from build123d import *

# Parameters (mm, degrees)
SKETCH_3_W             = 131
SKETCH_3_H             = 80
EXTRUDE_3_DEPTH        = 5
SKETCH_4_W             = 119
SKETCH_4_H             = 80
EXTRUDE_4_DEPTH        = 6
FILLET_2_R             = 5
CHAMFER_1_SIZE         = 1
CUT_EXTRUDE_1_DEPTH    = 6
FILLET_3_R             = 5
CHAMFER_2_SIZE         = 1
SKETCH_6_R             = 2.2
CUT_EXTRUDE_2_DEPTH    = 11
HOLE_WIZARD_M3_1_D     = 2.5
HOLE_WIZARD_M3_1_DEPTH = 7.5
HOLE_WIZARD_M3_1_TIP   = 0.751075774


with BuildPart() as part:
    # 草图3 → 凸台-拉伸3 (new body)
    with BuildSketch(Plane.XY):
        with Locations((0, -51.5)):
            Rectangle(SKETCH_3_W, SKETCH_3_H)
    extrude(amount=EXTRUDE_3_DEPTH)

    # 草图4 → 凸台-拉伸4 (add)
    with BuildSketch(Plane.XY.offset(5)):
        with Locations((0, -51.5)):
            Rectangle(SKETCH_4_W, SKETCH_4_H)
    extrude(amount=-EXTRUDE_4_DEPTH)

    # 圆角2
    fillet_2_edges = [part.edges().sort_by_distance(p)[0] for p in [
        (-65.5, -11.5, 2.5),
        (65.5, -11.5, 2.5),
        (65.5, -91.5, 2.5),
        (-65.5, -91.5, 2.5),
    ]]
    fillet(fillet_2_edges, radius=FILLET_2_R)

    # 倒角1
    chamfer_1_edges = [part.edges().sort_by_distance(p)[0] for p in [
        (0, -11.5, 5),
        (65.5, -51.5, 5),
        (0, -91.5, 5),
        (-65.5, -51.5, 5),
        (64.035533906, -90.035533906, 5),
        (-64.035533906, -90.035533906, 5),
        (-64.035533906, -12.964466094, 5),
        (64.035533906, -12.964466094, 5),
    ]]
    chamfer(chamfer_1_edges, length=CHAMFER_1_SIZE)

    # 草图5 → 切除-拉伸1 (cut)
    with BuildSketch(Plane.XY.offset(5)):
        Polygon((-10.644021059, -51.5), (-54.5, -28.163791023), (-54.5, -74.836208978), align=None)
        Polygon((43.855978941, -22.5), (-43.855978941, -22.5), (0, -45.836208978), align=None)
        Polygon((54.5, -28.163791023), (10.644021059, -51.5), (54.5, -74.836208978), align=None)
        Polygon((43.855978941, -80.5), (0, -57.163791023), (-43.855978941, -80.5), align=None)
    extrude(amount=-CUT_EXTRUDE_1_DEPTH, mode=Mode.SUBTRACT)

    # 圆角3
    fillet_3_edges = [part.edges().sort_by_distance(p)[0] for p in [
        (10.644021059, -51.5, 2),
        (54.5, -28.163791023, 2),
        (54.5, -74.836208978, 2),
        (-43.855978941, -22.5, 2),
        (43.855978941, -22.5, 2),
        (0, -45.836208978, 2),
        (-43.855978941, -80.5, 2),
        (0, -57.163791023, 2),
        (43.855978941, -80.5, 2),
        (-54.5, -74.836208978, 2),
        (-54.5, -28.163791023, 2),
        (-10.644021059, -51.5, 2),
    ]]
    fillet(fillet_3_edges, radius=FILLET_3_R)

    # 倒角2
    chamfer_2_edges = [part.edges().sort_by_distance(p)[0] for p in [
        (33.045284631, -39.580061586, 5),
        (54.5, -51.5, 5),
        (33.045284631, -63.419938415, 5),
        (14.256439507, -38.250213644, 5),
        (-14.256439507, -38.250213644, 5),
        (0, -22.5, 5),
        (-33.045284631, -39.580061586, 5),
        (-33.045284631, -63.419938415, 5),
        (-54.5, -51.5, 5),
        (-14.256439507, -64.749786356, 5),
        (14.256439507, -64.749786356, 5),
        (0, -80.5, 5),
        (52.074521107, -32.201893935, 5),
        (52.074521107, -70.798106066, 5),
        (16.288042118, -51.5, 5),
        (0, -45.172417956, 5),
        (-28.666695849, -26.289632976, 5),
        (28.666695849, -26.289632976, 5),
        (-16.288042118, -51.5, 5),
        (-52.074521107, -70.798106066, 5),
        (-52.074521107, -32.201893935, 5),
        (0, -57.827582045, 5),
        (28.666695849, -76.710367025, 5),
        (-28.666695849, -76.710367025, 5),
    ]]
    chamfer(chamfer_2_edges, length=CHAMFER_2_SIZE)

    # 草图6 → 切除-拉伸2 (cut)
    with BuildSketch(Plane.XY.offset(5)):
        with Locations(Location((62.5, -21.5, 0), (0, 0, 24.619977329))):
            Circle(SKETCH_6_R)
        with Locations(Location((62.5, -31.5, 0), (0, 0, 24.619977329))):
            Circle(SKETCH_6_R)
        with Locations(Location((62.5, -41.5, 0), (0, 0, 24.619977329))):
            Circle(SKETCH_6_R)
        with Locations(Location((62.5, -51.5, 0), (0, 0, 24.619977329))):
            Circle(SKETCH_6_R)
        with Locations(Location((62.5, -61.5, 0), (0, 0, 24.619977329))):
            Circle(SKETCH_6_R)
        with Locations(Location((62.5, -71.5, 0), (0, 0, 24.619977329))):
            Circle(SKETCH_6_R)
        with Locations(Location((62.5, -81.5, 0), (0, 0, 335.380022671))):
            Circle(SKETCH_6_R)
    cut_extrude_2 = extrude(amount=-CUT_EXTRUDE_2_DEPTH, mode=Mode.SUBTRACT)

    # 镜向1: 切除-拉伸2 across plane
    add(cut_extrude_2.mirror(Plane(origin=(0, 0, 0), x_dir=(0, 0, 1), z_dir=(1, 0, 0))), mode=Mode.SUBTRACT)

    # M3 螺纹孔1
    with Locations(Plane.XY.offset(5)):
        with Locations((-43.51, -20.75), (43.51, -20.75), (43.51, -80.29), (-43.51, -80.29)):
            Hole(HOLE_WIZARD_M3_1_D / 2, depth=HOLE_WIZARD_M3_1_DEPTH)
            with Locations((0, 0, -(HOLE_WIZARD_M3_1_DEPTH + HOLE_WIZARD_M3_1_TIP / 2))):  # 118° drill point
                Cone(0, HOLE_WIZARD_M3_1_D / 2, HOLE_WIZARD_M3_1_TIP, mode=Mode.SUBTRACT)


solid = part.part
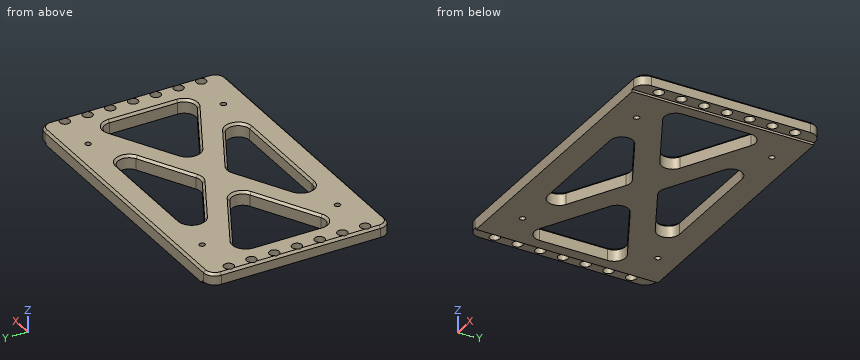
Build history of the part. All positions in model axes, mm. Coordinates: 2 decimals unless noted, no trailing zeros. Order: outer loops, then holes, each group sorted by start corner. A loop starts at its lowest first (then second) coordinate and runs counter-clockwise, first axis right, second up. Notation, with made-up numbers: (23.5, -17) - (60.5, -17) arc R27 cw to (60.5, 13) - close; hole circle Ø11 at (-16, -38.75). An arc over 180 degrees is marked (long way). Put each result on its own line as item: value.
1. Probe line 1 along X through (y, z) = (-51.5, 3.1); line 2 along Y through (x, z) = (43.5, -0.5); line 3 along X through (y, z) = (-66.5, 3.75). List the from-to ranges inside material, lowest first. Write a range as [from, to].
Answer sheet:
line 1: x = [-65.5, -64.7], [-60.3, -54.5], [-16.29, 16.29], [54.5, 60.3], [64.7, 65.5]
line 2: y = [-91.5, -81.54], [-79.04, -68.98], [-34.02, -22], [-19.5, -11.5]
line 3: x = [-65.5, -54.5], [-38.83, -17.55], [17.55, 38.83], [54.5, 65.5]
2. Saw through at C-C (z = 2). Give the number of separate pieces and of enclosed holes in the cut face, and give its area (3 significant figures).
Answer sheet:
separate pieces: 1
enclosed holes: 22
area: 6,510 mm^2
3. Drop a flat-ended pin along its axis: P1, Ø5, axis at x = -62.5, y = -71.5, coming from the -Z side. Give the stop position or say it passes through.
Answer sheet:
P1: stops at z = 0
4. Saw through at A-A (x = -38). Write the cut outline in (y, z).
Answer sheet:
outline: (-91.5, -1) - (-66.06, -1) - (-66.06, 4) - (-67.19, 5) - (-90.5, 5) - (-91.5, 4) - close; (-36.94, -1) - (-11.5, -1) - (-11.5, 4) - (-12.5, 5) - (-35.81, 5) - (-36.94, 4) - close
5. Saw through at B-B (x = 10.5). Write the cut outline in (y, z).
Answer sheet:
outline: (-91.5, -1) - (-80.5, -1) - (-80.5, 4) - (-81.5, 5) - (-90.5, 5) - (-91.5, 4) - close; (-62.75, -1) - (-40.25, -1) - (-40.25, 4) - (-41.38, 5) - (-61.62, 5) - (-62.75, 4) - close; (-22.5, -1) - (-11.5, -1) - (-11.5, 4) - (-12.5, 5) - (-21.5, 5) - (-22.5, 4) - close
